CAD build for the part. Positions are in the model's coordinates, mm. Give positions to 0.01 mm unless a question says otherwise; leave off trailing zeros. Loops run counter-clockwise (first coordinate to the right, second up) from the corner with the lowest first, then second, coordinate; pieces in that order, holes last. Notation, with made-up numbers: M -6.5,38 L 16.5,38 A33 cw 16.5,68 Z; hole C -24,63.25 d3. An arc over 180 degrees is marked long. One line per question, with ' | ' between items.
Autodesk Inventor part; units mm, degrees
ref_plane "YZ Plane" through (0, 0, 0) normal (1, 0, 0) x (0, 1, 0)
ref_plane "XZ Plane" through (0, 0, 0) normal (0, 1, 0) x (-1, 0, 0)
ref_plane "XY Plane" through (0, 0, 0) normal (0, 0, 1) x (1, 0, 0)
sketch "Sketch1" plane through (0, 0, 0) normal (0, 0, 1) x (1, 0, 0)
  line L0 (-33.6909, 31.0213) -> (-8.6909, 31.0213)
  line L1 (-8.6909, 31.0213) -> (-8.6909, 1.0213)
  line L2 (-8.6909, 1.0213) -> (-33.6909, 1.0213)
  line L3 (-33.6909, 1.0213) -> (-33.6909, 31.0213)
  circle A0 centre (-27.6909, 20.5213) radius 1.5
  circle A1 centre (-14.6909, 20.5213) radius 1.5
  line L4 (-21.1909, 1.0213) -> (-21.1909, 31.0213)
  line L5 (-33.6909, 16.0213) -> (-8.6909, 16.0213)
  dimension "d0" = 25
  dimension "d1" = 30
  dimension "d4" = 3
  dimension "d5" = 3
  dimension "d6" = 13
  dimension "d7" = 6
  dimension "d8" = 10.5
extrude "Extrusion1" add sketch "Sketch1" along normal blind 2
equation "\"d4\" = d5"
properties part number "Placa PCB 30x25"
Item 1: Mould opens along Y. For faces 1 (the flat face through (-21, 1.021, 1)), 2 (the flat face through (-21, 16, 2)), 3 (the cylindrical face through (-13.26, 20.07, 0.99)) say: pulls with the +Y half, pulls with the -Y half, needs draft (parallel to the pull), parting line crosses it, or undercut.
Conclusion:
face 1: pulls with the -Y half | face 2: needs draft | face 3: undercut
Item 2: Saw through at A-A on x = -28. Give the cut face in (y, z).
Conclusion:
outline: M 1.02,0 L 19.05,0 L 19.05,2 L 1.02,2 Z; M 21.99,0 L 31.02,0 L 31.02,2 L 21.99,2 Z
Item 3: Saw through at B-B on z = 0.9. Give the cut face in (x, y), and give its area (3 significant figures).
Conclusion:
outline: M -33.69,1.02 L -8.69,1.02 L -8.69,31.02 L -33.69,31.02 Z; hole C -27.69,20.52 d3; hole C -14.69,20.52 d3 | area: 736 mm²
Item 4: Drill centre lines: line 1 along X through (y, z) = (20.25, 0.7); line 2 along Y through (x, z) = (-15.75, 0.35); line 3 along Y through (x, z) = (-16, 0.25). Where is each one in solid material? Low to high. Write a range as [from, to].
Conclusion:
line 1: [-33.69, -29.17], [-26.22, -16.17], [-13.22, -8.69] | line 2: [1.02, 19.46], [21.58, 31.02] | line 3: [1.02, 19.79], [21.25, 31.02]
